Check sheet for the modelled part. Datum: model origin and axes. Units: mm. Round coordinates to 2 decimals unless told otherwise and drop trailing zeros. Loops run counter-clockwise (first coordinate to the right, second up) from the corner with the lowest first, then second, coordinate; pieces in that order, holes last. Notation, with made-up numbers: (-23, -18) - (6, -18) arc R26 cw to (6, -1) - close; hole circle Ø9 at (19, 57.25). An arc over 180 degrees is marked (long way). Answer in a Markdown table with one row per item. Add a question column.
(1) Thickness scan on line 1 along X through (y, z) = (423, 1.85); line 2 along X through (y, z) = (355, 0.95); line 3 along Y through (x, z) = (15.5, 2.5). Record the ranges inside material, lowest first.
(2) Gauge pin test, flat end, axial feed: pin 1 (1 mm diameter, centred on x = -10.5, z = 2.5, fed in from +Y). Record the tip position at first contact, or that the pin passes through.
(3) Cross-section at C-C on z = 3.85. Enter the section's corners in (x, y).
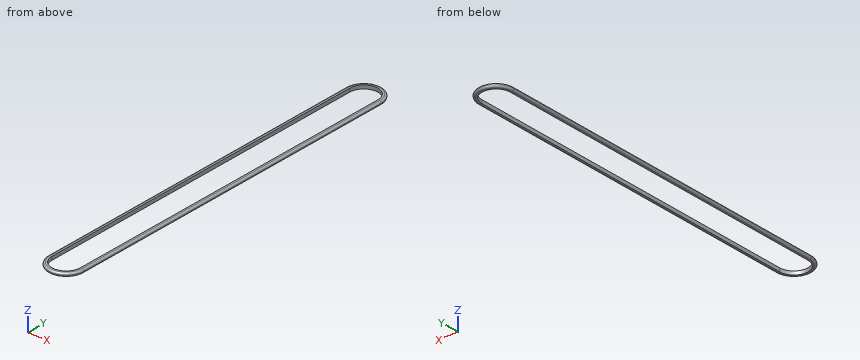
Autodesk Inventor part; units mm, degrees
ref_plane "YZ Plane" through (0, 0, 0) normal (1, 0, 0) x (0, 1, 0)
ref_plane "XZ Plane" through (0, 0, 0) normal (0, 1, 0) x (-1, 0, 0)
ref_plane "XY Plane" through (0, 0, 0) normal (0, 0, 1) x (1, 0, 0)
sketch "Sketch1" plane through (0, 0, 0) normal (0, 0, 1) x (1, 0, 0)
  arc A0 (-19.05, 0) -> (19.05, 0) centre (0, 0) ccw
  arc A1 (19.05, 469.9) -> (-19.05, 469.9) centre (0, 469.9) ccw
  line L0 (-19.05, 0) -> (-19.05, 469.9)
  line L1 (19.05, 469.9) -> (19.05, 0)
  arc A2 (23.8125, 469.9) -> (-23.8125, 469.9) centre (0, 469.9) ccw
  arc A3 (-23.8125, 0) -> (23.8125, 0) centre (0, 0) ccw
  line L2 (-23.8125, 469.9) -> (-23.8125, 0)
  line L3 (23.8125, 0) -> (23.8125, 469.9)
  dimension "d0" = 469.9
  dimension "d1" = 19.05
  dimension "d2" = 4.7625
extrude "Extrusion1" add sketch "Sketch1" along normal blind 4.7625
fillet "Fillet1" radius 2.3813 8 edges at (0, 493.7125, 4.7625) (23.8125, 234.95, 4.7625) (0, -23.8125, 4.7625) (-23.8125, 234.95, 4.7625) (0, -23.8125, 0) (23.8125, 234.95, 0) (0, 493.7125, 0) (-23.8125, 234.95, 0)
properties part number "Belt_VerticalConveyor_Rear"
Answers:
| question | item | result |
|---|---|---|
| 1 | line 1 | x = -23.75 to -19.05, 19.05 to 23.75 |
| 1 | line 2 | x = -23.33 to -19.05, 19.05 to 23.33 |
| 1 | line 3 | y = -18.07 to -11.07, 480.97 to 487.97 |
| 2 | pin 1 | stops at y = 491.51 |
| 3 | outline | (-23.31, 0) arc R23.31 ccw to (23.31, 0) - (23.31, 469.9) arc R23.31 ccw to (-23.31, 469.9) - close; hole (-19.05, 0) arc R19.05 ccw to (19.05, 0) - (19.05, 469.9) arc R19.05 ccw to (-19.05, 469.9) - close |
